Drawing for the job (mm, zero at the part's lowest x, y, z). A direction names the side the tool comes from. Round coordinates to 2 decimals unless told otherwise and drop trailing zeros. Write each loop counter-clockwise with the first axis right and the second up, starting at its lowest first coordinate (ties: lowest second). Pieces come first, ordered by that corner, then holes. Notation, with made-up numbers: M -10,0.25 L 33,0.25 A12 cw 33,23.25 Z; hole C -8,13.5 d11. An arc over 180 degrees is marked long. Use a Markdown table: item, result.
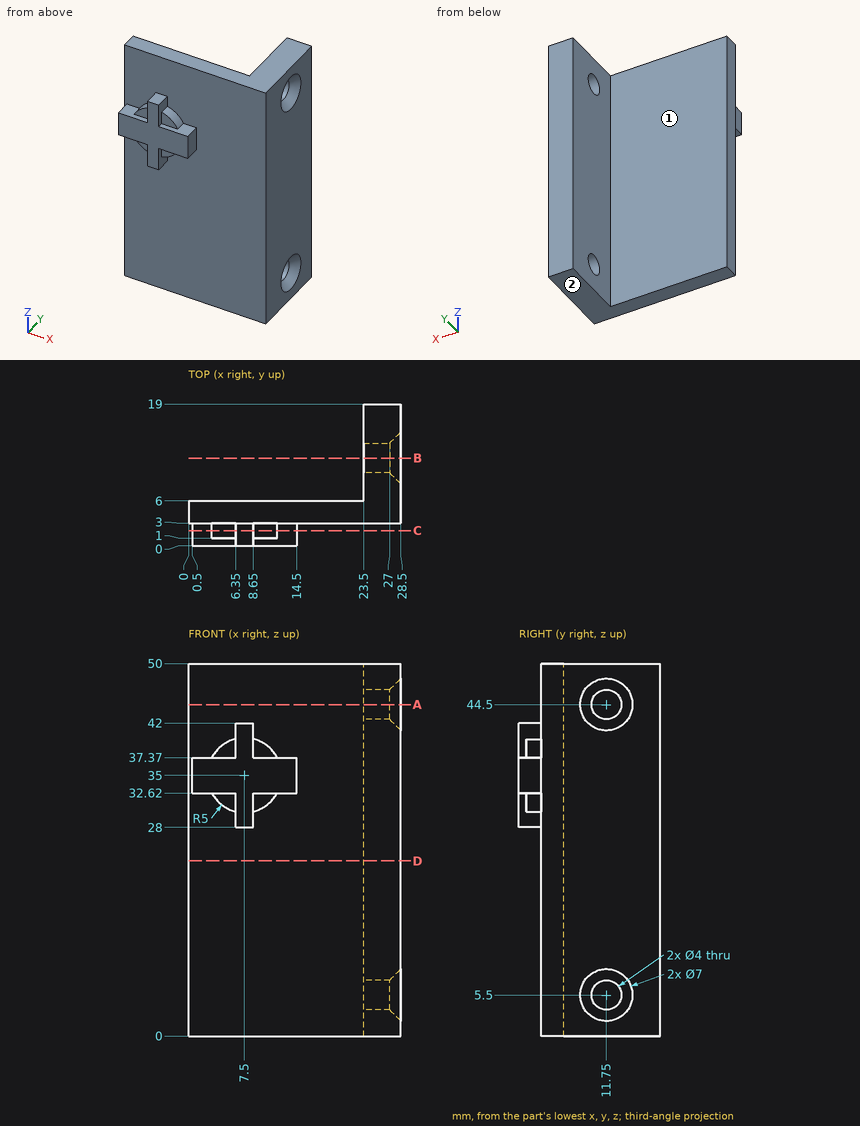
Q1. Cut at A-A on z = 44.5. Give the cut face in (x, y).
Response values:
| item | result |
|---|---|
| outline | M 0,3 L 28.5,3 L 28.5,8.25 L 27,9.75 L 23.5,9.75 L 23.5,6 L 0,6 Z; M 23.5,13.75 L 27,13.75 L 28.5,15.25 L 28.5,19 L 23.5,19 Z |
Q2. Cut at C-C on y = 2. Give the cut face in (x, z), and give its area (3 significant figures).
Response values:
| item | result |
|---|---|
| outline | M 0.5,32.62 L 3.1,32.62 A5 ccw 6.35,30.13 L 6.35,28 L 8.65,28 L 8.65,30.13 A5 ccw 11.9,32.62 L 14.5,32.62 L 14.5,37.37 L 11.9,37.37 A5 ccw 8.65,39.87 L 8.65,42 L 6.35,42 L 6.35,39.87 A5 ccw 3.1,37.37 L 0.5,37.37 Z |
| area | 109 mm2 |
Q3. Cut at B-B on y = 11.75. Give the cut face in (x, z).
Response values:
| item | result |
|---|---|
| outline | M 23.5,0 L 28.5,0 L 28.5,2 L 27,3.5 L 23.5,3.5 Z; M 23.5,7.5 L 27,7.5 L 28.5,9 L 28.5,41 L 27,42.5 L 23.5,42.5 Z; M 23.5,46.5 L 27,46.5 L 28.5,48 L 28.5,50 L 23.5,50 Z |
Q4. Drill centre lines: L1, parallel to Z at x = 25.5, y = 11.75; L2, parallel to Y at x = 25.15, z = 44.5; L3, parallel to X at y = 1.5, z = 35. Where is each one in solid material? Low to high.
Response values:
| item | result |
|---|---|
| L1 | z = 0 to 3.5, 7.5 to 42.5, 46.5 to 50 |
| L2 | y = 3 to 9.75, 13.75 to 19 |
| L3 | x = 0.5 to 14.5 |
Q5. Cut at D-D on z = 23.5. Give the cut face in (x, y), and give its area (4 significant figures).
Response values:
| item | result |
|---|---|
| outline | M 0,3 L 28.5,3 L 28.5,19 L 23.5,19 L 23.5,6 L 0,6 Z |
| area | 150.5 mm2 |
Q6. Which spindle directions (+Z, -Z, +X, -X, +Y, -Y) get a long thin tool onto all of the face, cutting with end or side? Do the marked faces 1 and 2. Say none if no direction does.
Response values:
| item | result |
|---|---|
| face 1 | +Z, -Z, -X, +Y |
| face 2 | -Z, +X, -X, +Y, -Y |
Q7. Drop flat-ended pins along their axis: P1, Ø3.5, axis at y = 1, z = 35.5, coming from the -X side; P2, Ø3, axis at y = 16, z = 42, coming from the -X side; P3, Ø1, axis at x = 4.5, z = 43, coming from the +Y side. Give the stop position or say it passes through.
Response values:
| item | result |
|---|---|
| P1 | stops at x = 0.5 |
| P2 | stops at x = 23.5 |
| P3 | stops at y = 6 |
